Geometry check sheet. Reference: the model listing, model coordinates, mm. Face numbers are marked on the shaded views. A direction names the side the tool comes from. Round coordinates to 2 decimals unless told otherwise and drop trailing zeros. Loops run counter-clockwise (first coordinate to the right, second up) from the corner with the lowest first, then second, coordinate; pieces in that order, holes last. Notation, with made-up numbers: (-3.5, 61) - (55.5, 61) arc R17 cw to (55.5, 78) - close; hole circle Ø5 at (73, 41). An arc over 180 degrees is marked (long way). Answer as CSV lines item,"result". Start each with the question number.
1) Thickness scan on line 1 along X through (y, z) = (-18.5, -45.5); line 2 along Z through (x, y) = (-9, -11.75); line 3 along Y through (x, z) = (33, -54.5). Record the ranges inside material, lowest first.
2) Access from +Z, -Z, +X, -X, +Y, -Y to the whole of each face (thin tool, end or side, straight path). Record for the marked faces 4 and 5.
3) Draft check along Z on the marked faces 1, 2 and 3. Enter one of: released by +Z, released by -Z, zero draft, split by the parting line, or undercut.
4) Cross-section at A-A on y = -18.5. Record the boundary of the cut face in (x, z).
5) Cross-section at B-B on x = 27. Record the boundary of the cut face in (y, z), and give its area (3 significant figures).
6) Depth check by flat-ended pin: P1, Ø2, axis at x = -6.5, y = -24, coming from the +Z side; P2, Ø6, axis at x = 10.5, z = -31.5, coming from the -Y side; P3, Ø2, axis at y = -24.5, z = 27.5, coming from the -X side. Enter the tip coordinate at first touch or a pass-through.
7) Cross-section at C-C on z = -3. Record the boundary of the cut face in (x, y).
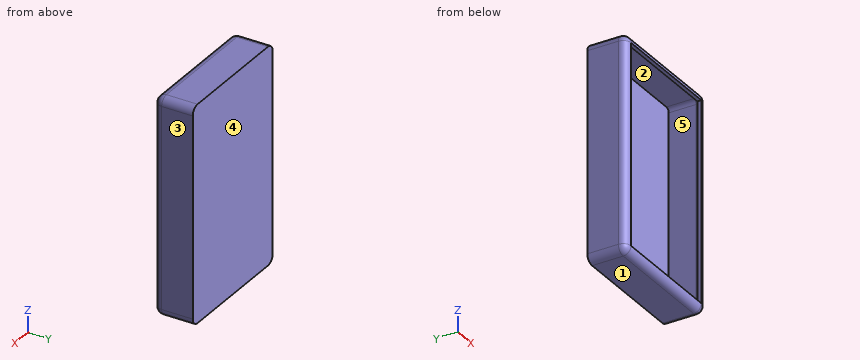
from build123d import *

# Parameters (mm, degrees)
F0_W     = 85.1108208299
F0_H     = 140.7826244831
F1_DEPTH = 25.4
F2_R     = 5.08
F3_T     = -2.54


# Not quite as in the source:
# - a shell that OpenCascade refuses in one call is made with other operations: the cavity is built on its own and cut out


with BuildPart() as f1:
    # F0 (on Front) → F1 (new body)
    with BuildSketch(Plane.XZ):
        Rectangle(F0_W, F0_H)
    extrude(amount=F1_DEPTH)

    # F2
    f2_edges = [f1.edges().sort_by_distance(p)[0] for p in [
        (0, -25.4, 70.391312),
        (-42.55541, -25.4, 0),
        (0, -25.4, -70.391312),
        (42.55541, -25.4, 0),
        (-42.55541, -12.7, 70.391312),
        (42.55541, -12.7, 70.391312),
        (-42.55541, -12.7, -70.391312),
        (42.55541, -12.7, -70.391312),
    ]]
    fillet(f2_edges, radius=F2_R)

    # F3: a shell. OpenCascade refuses it in one call, so the cavity is built on its own and cut out:
    # the body offset inwards by the wall thickness, plus a prism from it out through each open face.
    f3_core = offset(f1.part, amount=F3_T, mode=Mode.PRIVATE)
    f3_exits = [f3_core.faces().sort_by_distance(p)[0] for p in [
        (0, -22.86, 0),
    ]]
    add(f3_core, mode=Mode.SUBTRACT)
    extrude(f3_exits, amount=-F3_T, mode=Mode.SUBTRACT)


solid = f1.part
Answer block:
1,line 1,"x = -42.56 to -40.02, 40.02 to 42.56"
1,line 2,"z = -70.39 to -67.85, 67.85 to 70.39"
1,line 3,"y = -2.54 to 0"
2,face 4,"+Z, -Z, +X, -X, +Y"
2,face 5,"none"
3,face 1,"released by -Z"
3,face 2,"undercut"
3,face 3,"zero draft"
4,outline,"(-42.56, -65.31) arc R5.08 ccw to (-37.48, -70.39) - (37.48, -70.39) arc R5.08 ccw to (42.56, -65.31) - (42.56, 65.31) arc R5.08 ccw to (37.48, 70.39) - (-37.48, 70.39) arc R5.08 ccw to (-42.56, 65.31) - close; hole (-40.02, -65.31) arc R2.54 ccw to (-37.48, -67.85) - (37.48, -67.85) arc R2.54 ccw to (40.02, -65.31) - (40.02, 65.31) arc R2.54 ccw to (37.48, 67.85) - (-37.48, 67.85) arc R2.54 ccw to (-40.02, 65.31) - close"
5,outline,"(-25.4, -65.31) arc R5.08 ccw to (-20.32, -70.39) - (0, -70.39) - (0, 70.39) - (-20.32, 70.39) arc R5.08 ccw to (-25.4, 65.31) - (-22.86, 65.31) arc R2.54 cw to (-20.32, 67.85) - (-2.54, 67.85) - (-2.54, -67.85) - (-20.32, -67.85) arc R2.54 cw to (-22.86, -65.31) - close"
5,area,"478 mm^2"
6,P1,"stops at z = 69.63"
6,P2,"stops at y = -2.54"
6,P3,"stops at x = -41.44"
7,outline,"(-42.56, -20.32) arc R5.08 ccw to (-37.48, -25.4) - (-37.48, -22.86) arc R2.54 cw to (-40.02, -20.32) - (-40.02, -2.54) - (40.02, -2.54) - (40.02, -20.32) arc R2.54 cw to (37.48, -22.86) - (37.48, -25.4) arc R5.08 ccw to (42.56, -20.32) - (42.56, 0) - (-42.56, 0) - close"
